Part model, mm, in its own coordinate system. A direction names the side the tool comes from. Round coordinates to 2 decimals unless told otherwise and drop trailing zeros. Write each loop counter-clockwise with the first axis right and the second up, starting at its lowest first coordinate (ties: lowest second). Pieces come first, ordered by that corner, then holes. Notation, with made-up numbers: M 65.5,14 L 119.5,14 A23 ccw 119.5,34 Z; hole C 66,56 d6. An arc over 180 degrees is marked long. Use a Markdown table: item, result. Add a question column.
1) Slice it at C-C on y = 15.5. Write the cut outline in (x, z) (3 decimals), plus the area to 3 significant figures.
2) Slice it at B-B on y = -9. Write the cut outline in (x, z).
3) Which spindle directions (+Z, -Z, +X, -X, +Y, -Y) get a long thin tool onto all of the face, cutting with end or side? Do faces 1 (the face through (-0.97, -14.72, 5.27)), 2 (the face through (15, -12.45, 7)), 3 (the face through (-13.253, 31.492, 4.056)), 4 (the face through (-7.5, -25, 4)), 5 (the face through (-15, -30, 4)). Say none if no direction does.
4) Wall check: probe 1 along Y at (x, z) = (1, 1.5); probe 2 along Y at (x, z) = (15, 3); probe 3 along X at (y, z) = (-19.3, 4). Give the ranges that are in metal, low to high.
5) Slice it at A-A on x = 0. Write the cut outline in (y, z), plus the area to 3 significant figures.
6) Slice it at D-D on z = 4. Give the number of separate pieces and of enclosed holes in the cut face, plus the area to 3 significant figures.
7) Drop flat-ended pins along their axis: P1, Ø1.6, axis at x = 29, z = 3.5, coming from the +Y side; P2, Ø4.5, axis at x = 29.5, z = 4.5, coming from the +Y side; P3, Ø1, axis at y = 23.5, z = 2.5, coming from the -X side. Give the stop position or say it passes through.
8) Two-plate mould, pull along Y, no slides. Class faces 6 (the face through (-20.074, 15.433, 6.521)), 7 (the face through (-21, -29, 4)), 8 (the face through (47.668, 27.436, 3.944)): released by +Y, released by -Y, zero draft, split by the parting line, or undercut.
```python
from build123d import *

# Parameters (mm, degrees)
SKETCH_3_R          = 4.05
SKETCH_3_W          = 6.1
SKETCH_3_H          = 3
EXTRUDE_1_DEPTH     = 8
CUT_EXTRUDE_2_DEPTH = 3
SKETCH_6_R          = 1.6
CUT_EXTRUDE_3_DEPTH = 15
SKETCH_7_R          = 4.05
CUT_EXTRUDE_4_DEPTH = 68.662198854
CHAMFER_1_SIZE      = 2
EXTRUDE_2_DEPTH     = 8


with BuildPart() as part:
    # 草图3 → 凸台-拉伸1 (new body)
    with BuildSketch(Plane.XY):
        with BuildLine():
            Line((43.971143614, 31.160253781), (20.588455044, 44.660256921))
            ThreePointArc((20.588455044, 44.660256921), (18.176645298, 45.659261336), (15.5884546, 46.000003139))
            Line((15.5884546, 46.000003139), (-7.779942733, 46.000003139))
            ThreePointArc((-7.779942733, 46.000003139), (-22.764282879, 39.246495142), (-27.628936924, 23.546958177))
            Line((-27.628936924, 23.546958177), (-25.213219189, 4))
            Line((-25.213219189, 4), (-13.416407865, 4))
            ThreePointArc((-13.416407865, 4), (14, 0), (-13.416407865, -4))
            Line((-13.416407865, -4), (-24.224536362, -4))
            Line((-24.224536362, -4), (-22, -22))
            Line((-22, -22), (-22, -30))
            Line((-22, -30), (-7.5, -30))
            Line((-7.5, -30), (-7.5, -22))
            Line((-7.5, -22), (33.97114317, -22))
            Line((33.97114317, -22), (33.97114317, -30))
            Line((33.97114317, -30), (48.97114317, -30))
            Line((48.97114317, -30), (48.97114317, 22.5))
            ThreePointArc((48.97114317, 22.5), (47.631397336, 27.499999778), (43.971143614, 31.160253781))
        make_face()
        with Locations((38.97114317, 22.5)):
            Circle(SKETCH_3_R, mode=Mode.SUBTRACT)
        with Locations((0, -17)):
            Rectangle(SKETCH_3_W, SKETCH_3_H, mode=Mode.SUBTRACT)
        with BuildLine():
            Line((-16.3, 17.1), (-14.7, 17.1))
            ThreePointArc((-14.7, 17.1), (-13.1, 15.5), (-14.7, 13.9))
            Line((-14.7, 13.9), (-16.3, 13.9))
            ThreePointArc((-16.3, 13.9), (-17.9, 15.5), (-16.3, 17.1))
        make_face(mode=Mode.SUBTRACT)
        with BuildLine():
            Line((14.7, 17.1), (16.3, 17.1))
            ThreePointArc((16.3, 17.1), (17.9, 15.5), (16.3, 13.9))
            Line((16.3, 13.9), (14.7, 13.9))
            ThreePointArc((14.7, 13.9), (13.1, 15.5), (14.7, 17.1))
        make_face(mode=Mode.SUBTRACT)
        with BuildLine():
            Line((14.7, -13.9), (16.3, -13.9))
            ThreePointArc((16.3, -13.9), (17.9, -15.5), (16.3, -17.1))
            Line((16.3, -17.1), (14.7, -17.1))
            ThreePointArc((14.7, -17.1), (13.1, -15.5), (14.7, -13.9))
        make_face(mode=Mode.SUBTRACT)
        with BuildLine():
            Line((-16.3, -13.9), (-14.7, -13.9))
            ThreePointArc((-14.7, -13.9), (-13.1, -15.5), (-14.7, -17.1))
            Line((-14.7, -17.1), (-16.3, -17.1))
            ThreePointArc((-16.3, -17.1), (-17.9, -15.5), (-16.3, -13.9))
        make_face(mode=Mode.SUBTRACT)
        with Locations((28.97114317, -17)):
            Rectangle(SKETCH_3_W, SKETCH_3_H, mode=Mode.SUBTRACT)
    extrude(amount=EXTRUDE_1_DEPTH)

    # 草图5 → 切除-拉伸2 (cut)
    with BuildSketch(Plane.XY.offset(8)):
        with BuildLine():
            Line((-17.025, 18.55), (-13.975, 18.55))
            ThreePointArc((-13.975, 18.55), (-10.925, 15.5), (-13.975, 12.45))
            Line((-13.975, 12.45), (-17.025, 12.45))
            ThreePointArc((-17.025, 12.45), (-20.075, 15.5), (-17.025, 18.55))
        make_face()
        with BuildLine():
            Line((13.975, 18.55), (17.025, 18.55))
            ThreePointArc((17.025, 18.55), (20.075, 15.5), (17.025, 12.45))
            Line((17.025, 12.45), (13.975, 12.45))
            ThreePointArc((13.975, 12.45), (10.925, 15.5), (13.975, 18.55))
        make_face()
        with BuildLine():
            Line((13.975, -12.45), (17.025, -12.45))
            ThreePointArc((17.025, -12.45), (20.075, -15.5), (17.025, -18.55))
            Line((17.025, -18.55), (13.975, -18.55))
            ThreePointArc((13.975, -18.55), (10.925, -15.5), (13.975, -12.45))
        make_face()
        with BuildLine():
            Line((-17.025, -12.45), (-13.975, -12.45))
            ThreePointArc((-13.975, -12.45), (-10.925, -15.5), (-13.975, -18.55))
            Line((-13.975, -18.55), (-17.025, -18.55))
            ThreePointArc((-17.025, -18.55), (-20.075, -15.5), (-17.025, -12.45))
        make_face()
    extrude(amount=-CUT_EXTRUDE_2_DEPTH, mode=Mode.SUBTRACT)

    # 草图6 → 切除-拉伸3 (cut)
    with BuildSketch(Plane.XZ.offset(22)):
        with Locations(Location((0, 4, 0), (0, 0, 270))):
            Circle(SKETCH_6_R)
        with Locations(Location((28.97114317, 4, 0), (0, 0, 270))):
            Circle(SKETCH_6_R)
    extrude(amount=-CUT_EXTRUDE_3_DEPTH, mode=Mode.SUBTRACT)

    # 草图7 → 切除-拉伸4 (cut, through all)
    with BuildSketch(Plane.XY.offset(8)):
        with Locations((38.97114317, 22.5)):
            Circle(SKETCH_7_R)
        with BuildLine():
            Line((-9.216024373, 24.574816528), (-5.72042198, 33.943955438))
            ThreePointArc((-5.72042198, 33.943955438), (-3.469092252, 34.971824328), (-2.441223361, 32.7204946))
            Line((-2.441223361, 32.7204946), (-5.936825754, 23.35135569))
            ThreePointArc((-5.936825754, 23.35135569), (-8.188156015, 22.323485372), (-9.216024373, 24.574816528))
        make_face()
        with BuildLine():
            Line((-18.304089115, 27.965550849), (-14.808486722, 37.334689759))
            ThreePointArc((-14.808486722, 37.334689759), (-12.557156994, 38.362558649), (-11.529288104, 36.111228921))
            Line((-11.529288104, 36.111228921), (-15.024890497, 26.742090011))
            ThreePointArc((-15.024890497, 26.742090011), (-17.276220757, 25.714219693), (-18.304089115, 27.965550849))
        make_face()
    extrude(amount=-CUT_EXTRUDE_4_DEPTH, mode=Mode.SUBTRACT)

    # 倒角1
    chamfer_1_edges = [part.edges().sort_by_distance(p)[0] for p in [
        (48.97114317, -30, 4),
        (33.97114317, -30, 4),
        (-7.5, -30, 4),
        (-22, -30, 4),
    ]]
    chamfer(chamfer_1_edges, length=CHAMFER_1_SIZE)

    # 草图8 → 凸台-拉伸2 (add)
    with BuildSketch(Plane.XY.offset(8)):
        Polygon((25.92114317, -15.5), (25.92114317, -18.5), (26.12114317, -18.5), (26.12114317, -15.9), (31.82114317, -15.9), (31.82114317, -18.5), (32.02114317, -18.5), (32.02114317, -15.5), align=None)
        Polygon((-2.85, -18.5), (-2.85, -15.9), (2.85, -15.9), (2.85, -18.5), (3.05, -18.5), (3.05, -15.5), (-3.05, -15.5), (-3.05, -18.5), align=None)
    extrude(amount=-EXTRUDE_2_DEPTH)


solid = part.part
```
Entries:
| question | item | result |
|---|---|---|
| 1 | outline | M -26.634,0 L -17.9,0 L -17.9,5 L -20.075,5 L -20.075,8 L -26.634,8 Z; M -13.1,0 L 13.1,0 L 13.1,5 L 10.925,5 L 10.925,8 L -10.925,8 L -10.925,5 L -13.1,5 Z; M 17.9,0 L 48.971,0 L 48.971,8 L 20.075,8 L 20.075,5 L 17.9,5 Z |
| 1 | area | 502 mm^2 |
| 2 | outline | M -23.61,0 L -10.72,0 L -10.72,8 L -23.61,8 Z; M 10.72,0 L 48.97,0 L 48.97,8 L 10.72,8 Z; hole C 28.97,4 d3.2 |
| 3 | face 1 | none |
| 3 | face 2 | +Z |
| 3 | face 3 | +Z, -Z |
| 3 | face 4 | +Z, -Z, -Y |
| 3 | face 5 | +Z, -Z, +X, -X, -Y |
| 4 | probe 1 | y = -22 to -18.5, -15.9 to -13.96, 13.96 to 46 |
| 4 | probe 2 | y = -22 to -17.1, -13.9 to 13.9, 17.1 to 46 |
| 4 | probe 3 | x = -22.33 to -1.6, 1.6 to 27.37, 30.57 to 48.97 |
| 5 | outline | M -22,0 L -18.5,0 L -18.5,2.4 L -22,2.4 Z; M -22,5.6 L -18.5,5.6 L -18.5,8 L -22,8 Z; M -15.9,0 L -14,0 L -14,2.4 L -15.5,2.4 L -15.5,5.6 L -14,5.6 L -14,8 L -15.9,8 Z; M 14,0 L 46,0 L 46,8 L 14,8 Z |
| 5 | area | 283 mm^2 |
| 6 | separate pieces | 1 |
| 6 | enclosed holes | 8 |
| 6 | area | 3,970 mm^2 |
| 7 | P1 | stops at y = 40.27 |
| 7 | P2 | stops at y = 40.81 |
| 7 | P3 | stops at x = -27.68 |
| 8 | face 6 | undercut |
| 8 | face 7 | released by -Y |
| 8 | face 8 | released by +Y |
